from build123d import *

# Parameters (mm, degrees)
F1_DEPTH = 64
F2_R     = 7
F3_DEPTH = 14


with BuildPart() as f1:
    # F0 (on Front) → F1 (new body)
    with BuildSketch(Plane.XZ):
        with BuildLine():
            Line((-44.4183332533, 0), (-34, 0))
            Line((-34, 0), (-23.7819293264, 0))
            ThreePointArc((-23.7819293264, 0), (-13, 7.5), (-2.2180706736, 0))
            ThreePointArc((-2.2180706736, 0), (-1.1090353368, -0.4900293956), (0, 0))
            ThreePointArc((0, 0), (0.1576676396, 1.9388564323), (0, 3.8777128647))
            ThreePointArc((0, 3.8777128647), (-3.676919168, 10.7323783319), (-10.7847960107, 13.8921663032))
            Line((-10.7847960107, 13.8921663032), (-12.8998687101, 13.8921663032))
            Line((-12.8998687101, 13.8921663032), (-13, 13.8921663032))
            Line((-13, 13.8921663032), (-55.1001312899, 13.8921663032))
            Line((-55.1001312899, 13.8921663032), (-57.2152039893, 13.8921663032))
            ThreePointArc((-57.2152039893, 13.8921663032), (-65.6365770881, 9.2975435208), (-68, 0))
            ThreePointArc((-68, 0), (-66.8909646632, -0.4900293956), (-65.7819293264, 0))
            ThreePointArc((-65.7819293264, 0), (-55.1001312899, 7.3366019369), (-44.4183332533, 0))
        make_face()
    extrude(amount=F1_DEPTH)

    # F2 (on Top) → F3 (cut)
    with BuildSketch(Plane.XY):
        with Locations((-34, -48)):
            Circle(F2_R)
        with BuildLine():
            ThreePointArc((-27, -16), (-29.0502525317, -11.0502525317), (-34, -9))
            Line((-34, -9), (-34, -23))
            ThreePointArc((-34, -23), (-29.0502525317, -20.9497474683), (-27, -16))
        make_face()
        with BuildLine():
            Line((-34, -23), (-34, -9))
            ThreePointArc((-34, -9), (-41, -16), (-34, -23))
        make_face()
    extrude(amount=F3_DEPTH, mode=Mode.SUBTRACT)


solid = f1.part
Work out the finished part from the listing and answer in its coordinate system (mm). A direction names the side the tool comes from. Round coordinates to 2 decimals unless told otherwise and drop trailing zeros. Write each loop counter-clockwise with the first axis right and the second up, starting at its lowest first coordinate (ties: lowest second). Pieces come first, ordered by that corner, then holes. Notation, with made-up numbers: (47, 82) -> (64, 82) arc R18 cw to (64, 112) -> close; hole circle Ø4 at (29.25, 57.5). An arc over 180 degrees is marked (long way). Answer as CSV lines item,"result". Start each with the question number.
(1) The part is cut by section B-B, the plane z = 2.25. Give the vertices of the cut face in (x, y).
(2) A tool of negligible diameter and unlimited length cuts with its end or side. For faces 4 (the flat face through (-34, -32, 0)), 5 (the cylindrical face through (-30.237, -42.098, 6.849)), from which of +Z, -Z, +X, -X, +Y, -Y can it reach the whole face along a straight path? Write none if from no direction.
(3) Each of these flat-tipped pins is pushed along its axis until it touches: pin 1 (4 mm diameter, centred on y = -31.5, z = 9.5, fed in from -X); pin 2 (5 mm diameter, centred on y = -35.5, z = 8.5, fed in from -X); pin 3 (3 mm diameter, centred on y = -24, z = 10, fed in from -X). Where does it stop, or does it pass through?
(4) The mould has two halves that part along X. Classify faces 1 (the flat face through (-34, 0, 8)), 2 (the cylindrical face through (-1.13, -31.55, -0.49)), 3 (the cylindrical face through (-65.55, -31.55, 9.41)): +X half, -X half, draft (parallel to the pull), parting line (faces both ways), or undercut.
(5) Find the intervals of material crossed by probe 1 along Y at (x, z) = (-34, 3.75); probe 2 along X at (y, z) = (-36.5, 2.25); probe 3 along Y at (x, z) = (-39, 1.5), in increasing order.
(6) The part is cut by section D-D, the plane y = -29.5. Give the vertices of the cut face in (x, z), then the cut area to 3 significant figures.
(7) The part is cut by section A-A, the plane y = -48. Give the vertices of the cut face in (x, z).
(8) The part is cut by section C-C, the plane x = -28.5. Give the vertices of the cut face in (y, z), then the cut area to 3 significant figures.
Output values:
1,outline,"(-68.15, -64) -> (-64.62, -64) -> (-64.62, 0) -> (-68.15, 0) -> close; (-45.58, -64) -> (-22.65, -64) -> (-22.65, 0) -> (-45.58, 0) -> close; (-3.35, -64) -> (0.15, -64) -> (0.15, 0) -> (-3.35, 0) -> close; hole circle Ø14 at (-34, -48); hole circle Ø14 at (-34, -16)"
2,face 4,"-Z, +Y, -Y"
2,face 5,"+Z, -Z"
3,pin 1,"stops at x = -66.79"
3,pin 2,"stops at x = -67.45"
3,pin 3,"stops at x = -66.21"
4,face 1,"draft"
4,face 2,"undercut"
4,face 3,"-X half"
5,probe 1,"y = -64 to -55, -41 to -23, -9 to 0"
5,probe 2,"x = -68.15 to -64.62, -45.58 to -22.65, -3.35 to 0.15"
5,probe 3,"y = -64 to -52.9, -43.1 to -20.9, -11.1 to 0"
6,outline,"(-68, 0) arc R1.5 ccw to (-65.78, 0) arc R11.44 cw to (-44.42, 0) -> (-23.78, 0) arc R11.5 cw to (-2.22, 0) arc R1.5 ccw to (0, 0) arc R12 ccw to (-10.78, 13.89) -> (-57.22, 13.89) arc R12 ccw to start"
6,area,"658 mm²"
7,outline,"(-68, 0) arc R1.5 ccw to (-65.78, 0) arc R11.44 cw to (-44.42, 0) -> (-41, 0) -> (-41, 13.89) -> (-57.22, 13.89) arc R12 ccw to start; (-27, 0) -> (-23.78, 0) arc R11.5 cw to (-2.22, 0) arc R1.5 ccw to (0, 0) arc R12 ccw to (-10.78, 13.89) -> (-27, 13.89) -> close"
8,outline,"(-64, 0) -> (-52.33, 0) -> (-52.33, 13.89) -> (-64, 13.89) -> close; (-43.67, 0) -> (-20.33, 0) -> (-20.33, 13.89) -> (-43.67, 13.89) -> close; (-11.67, 0) -> (0, 0) -> (0, 13.89) -> (-11.67, 13.89) -> close"
8,area,"648 mm²"
